For this review, take the finished solid that the model builds, in its own axes (mm). A direction names the side the tool comes from. Coordinates: 2 decimals unless noted, no trailing zeros. Loops run counter-clockwise (first coordinate to the right, second up) from the corner with the lowest first, then second, coordinate; pieces in that order, holes last. Notation, with made-up numbers: M 17.5,22 L 45.5,22 A32 ccw 45.5,61 Z; hole C 52.25,87 d9. An arc over 180 degrees is marked long. Use one line per item in the form item = value.
```python
from build123d import *

# Parameters (mm, degrees)
F0_R     = 2.25
F0_W     = 16
F0_H     = 6
F1_DEPTH = 1.5
F2_R     = 1
F3_R     = 2


with BuildPart() as f1:
    # F0 (on Top) → F1 (new body)
    with BuildSketch(Plane.XY):
        with BuildLine():
            Line((-25, -5), (11, -5))
            ThreePointArc((11, -5), (11.707107, -4.707107), (12, -4))
            Line((12, -4), (12, -3))
            Line((12, -3), (12, 3))
            Line((12, 3), (12, 5))
            Line((12, 5), (-25, 5))
            ThreePointArc((-25, 5), (-27.12132, 4.12132), (-28, 2))
            Line((-28, 2), (-28, -2))
            ThreePointArc((-28, -2), (-27.12132, -4.12132), (-25, -5))
        make_face()
        with Locations((-22.75, 0)):
            Circle(F0_R, mode=Mode.SUBTRACT)
        with Locations((20, 0)):
            Rectangle(F0_W, F0_H)
    extrude(amount=F1_DEPTH)

    # F2
    f2_edges = [f1.edges().sort_by_distance(p)[0] for p in [
        (12, 5, 0.75),
    ]]
    fillet(f2_edges, radius=F2_R)

    # F3
    f3_edges = [f1.edges().sort_by_distance(p)[0] for p in [
        (28, 3, 0.75),
        (28, -3, 0.75),
    ]]
    fillet(f3_edges, radius=F3_R)


solid = f1.part
```
1. Consider section B-B on y = 0. Write out the cut boundary in (x, z).
Computed values:
outline = M -28,0 L -25,0 L -25,1.5 L -28,1.5 Z; M -20.5,0 L 28,0 L 28,1.5 L -20.5,1.5 Z
2. Consider section A-A on x = -22.75. Write out the cut boundary in (y, z).
Computed values:
outline = M -5,0 L -2.25,0 L -2.25,1.5 L -5,1.5 Z; M 2.25,0 L 5,0 L 5,1.5 L 2.25,1.5 Z
3. For pin 1 Ø4 at (x, y) = (-22.75, 0) entering from +Z; pin 2 Ø0.8 at (y, z) = (-3.5, 0.5) entering from +X, all flat-tipped, find the tip position at first contact; note any pin that passes through.
Computed values:
pin_1 = through
pin_2 = 12
4. Consider section D-D on x = 13.5. Write out the cut boundary in (y, z), plus the area to 3 significant figures.
Computed values:
outline = M -3,0 L 3,0 L 3,1.5 L -3,1.5 Z
area = 9.00 mm2
5. Draft analysis for pull direction X (two halves, no side actions). For faces 4 (the face through (-20.604, 0.676, 0.74)), 5 (the face through (-27.1, 4.14, 0.74)), 6 (the face through (-7, 0, 1.5)), 7 (the face through (28, 0, 1)), state which applies: +X half, -X half, draft (parallel to the pull), parting line (faces both ways), or undercut.
Computed values:
face_4 = undercut
face_5 = -X half
face_6 = draft
face_7 = +X half
6. Wall thickness on line 1 along Y through (x, z) = (-22.75, 0.65); line 2 along Y through (x, z) = (23.5, 0.5); line 3 along X through (y, z) = (-3.75, 1.35): over which ranges is each line inside the solid? List them lowest first. Write a range as from..to.
Computed values:
line_1 = -5..-2.25, 2.25..5
line_2 = -3..3
line_3 = -27.44..12
7. Consider section C-C on z = 0.3. Write out the cut boundary in (x, y), plus the area to 3 significant figures.
Computed values:
outline = M -28,-2 A3 ccw -25,-5 L 11,-5 A1 ccw 12,-4 L 12,-3 L 26,-3 A2 ccw 28,-1 L 28,1 A2 ccw 26,3 L 12,3 L 12,4 A1 ccw 11,5 L -25,5 A3 ccw -28,2 Z; hole C -22.75,0 d4.5
area = 474 mm2
8. Tool access review of faces 1 (the face through (12, -3.5, 0.7)), 2 (the face through (19, 3, 1)), 3 (the face through (-7, 0, 0)): name each direction out of +Z, -Z, +X, -X, +Y, -Y from which nothing blocks a thin tool from reaching the whole face with its end or side.
Computed values:
face_1 = +Z, -Z, +X, -Y
face_2 = +Z, -Z, +X, +Y
face_3 = -Z, +X, -X, +Y, -Y
